Could you check a few things on this model? Use its own coordinates, in mm. Round coordinates to 2 decimals unless told otherwise and drop trailing zeros. Write each loop counter-clockwise with the first axis right and the second up, starting at its lowest first coordinate (ties: lowest second). Pieces come first, ordered by that corner, then holes. Notation, with made-up numbers: (89.25, -18) - (148.25, -18) arc R19 ccw to (148.25, 10) - close; hole circle Ø6 at (46.5, 21.5). An arc over 180 degrees is marked (long way). Put each result on its own line as item: value.
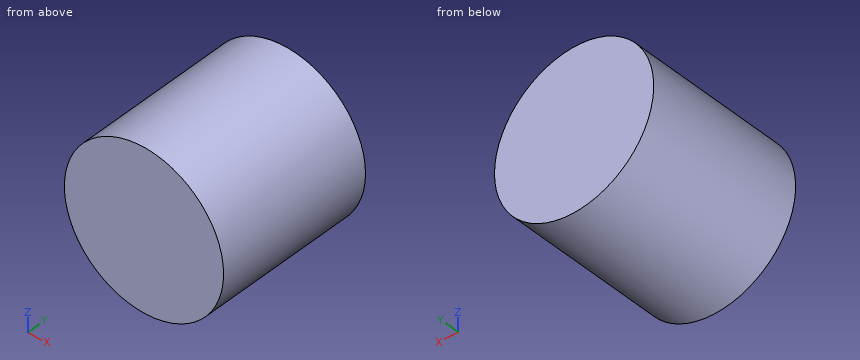
from build123d import *

# Parameters (mm, degrees)
F0_R      = 50.354649
F1_DEPTH  = 50.8
F3_DEPTH  = 25.4
F4_DEPTH  = 25.4
F1_FACE_R = 50.354649
F5_DEPTH  = 50.8


with BuildPart() as f1:
    # F0 (on Front) → F1 (new body)
    with BuildSketch(Plane.XZ):
        Circle(F0_R)
    extrude(amount=F1_DEPTH)

    # F2 (on Front) → F3 (join)
    with BuildSketch(Plane.XZ):
        Polygon((0, 0), (-25.05855, 43.402681), (-50.1171, 0), align=None)
        Polygon((25.05855, 43.402681), (-25.05855, 43.402681), (0, 0), align=None)
        Polygon((50.1171, 0), (25.05855, 43.402681), (0, 0), align=None)
        Polygon((0, 0), (-50.1171, 0), (-25.05855, -43.402681), align=None)
        Polygon((50.1171, 0), (0, 0), (25.05855, -43.402681), align=None)
        Polygon((25.05855, -43.402681), (0, 0), (-25.05855, -43.402681), align=None)
    extrude(amount=F3_DEPTH)

    # F2 (on Front) → F4 (join)
    with BuildSketch(Plane.XZ):
        Polygon((0, 0), (-25.05855, 43.402681), (-50.1171, 0), align=None)
        Polygon((25.05855, 43.402681), (-25.05855, 43.402681), (0, 0), align=None)
        Polygon((50.1171, 0), (25.05855, 43.402681), (0, 0), align=None)
        Polygon((0, 0), (-50.1171, 0), (-25.05855, -43.402681), align=None)
        Polygon((50.1171, 0), (0, 0), (25.05855, -43.402681), align=None)
        Polygon((25.05855, -43.402681), (0, 0), (-25.05855, -43.402681), align=None)
    extrude(amount=F4_DEPTH)

    # F1_face (on face) → F5 (join)
    with BuildSketch(Plane.XZ.offset(50.8)):
        Circle(F1_FACE_R)
    extrude(amount=F5_DEPTH)


solid = f1.part
(1) Imagine slicing it at A-A, the plane y = -19. List the corners of the cut face in (x, z) for me, then the cut area to 3 significant figures.
Values found:
outline: circle Ø100.71 at (0, 0)
area: 7,970 mm^2
(2) I'm going to push flat-ended pins straight in: pin 1 (8 mm diameter, centred on y = -50, z = 17, fed in from -X); pin 2 (12 mm diameter, centred on x = -19.5, y = -71, fed in from -Z); pin 3 (1 mm diameter, centred on x = -32.5, y = -42, fed in from +Z). Where does each tip first touch, or does it pass through?
Values found:
pin 1: stops at x = -48.65
pin 2: stops at z = -48.51
pin 3: stops at z = 38.88
(3) Please list where these lines run through material, in increasing order: probe 1 along Z at (x, y) = (46.5, -36); probe 2 along X at (y, z) = (-37.5, -27); probe 3 along X at (y, z) = (-43, 0.5). Write a range as from..to.
Values found:
probe 1: z = -19.32..19.32
probe 2: x = -42.5..42.5
probe 3: x = -50.35..50.35
(4) Imagine slicing it at B-B, the plane z = 29. List the corners of the cut face in (x, y) for me.
Values found:
outline: (-41.17, -101.6) - (41.17, -101.6) - (41.17, 0) - (-41.17, 0) - close
(5) Imagine slicing it at C-C, the plane x = 10. List the corners of the cut face in (y, z) for me.
Values found:
outline: (-101.6, -49.35) - (0, -49.35) - (0, 49.35) - (-101.6, 49.35) - close
